For this review, take the finished solid that the model builds, in its own axes (mm). A direction names the side the tool comes from. Coordinates: 2 decimals unless noted, no trailing zeros. Loops run counter-clockwise (first coordinate to the right, second up) from the corner with the lowest first, then second, coordinate; pieces in that order, holes last. Notation, with made-up numbers: (-22, 37) - (26, 37) arc R27 ccw to (26, 69) - close; hole circle Ø3 at (57.25, 72.25). An arc over 180 degrees is marked (long way). Answer as a JSON object with one key per item and string values. Group by question number.
Item 1: We need section C-C (x = 9). Give the boundary of the cut face in (y, z) (3 decimals).
Item 2: Tool access review of faces 5 (the cylindrical face through (4.97, -8.45, -11.02)), 6 (the cylindrical face through (0.74, 17.06, 10.88)), 7 (the flat face through (0, -4, 0)), 8 (the cylindrical face through (8.028, 12.118, 3.816)), 9 (the cylindrical face through (2, -5, 0)): name each direction out of +Z, -Z, +X, -X, +Y, -Y from which nothing blocks a thin tool from reaching the whole face with its end or side.
Item 3: Mouldability with a two-part tool opening along Y and no side actions: class faces 1 (the cylindrical face through (5, 0, 11)), 2 (the cylindrical face through (2.218, 0.867, -12.905)), 3 (the flat face through (10, -13, 0)), 4 (the conical face through (6.874, -13.856, -3.077)) as released by +Y, released by -Y, zero draft, split by the parting line, or undercut.
Item 4: To check wall thickness, follow line 1 (X direction, y = 9, z = 4.5); line 2 (Y direction, x = 9.25, z = 10.5); line 3 (X direction, y = 4, z = -14). State the ranges of each line that lie inside material, in increasing order.
Item 5: Clearance check with flat-ended pins moving along their axes: pin 1 (7 mm diameter, centred on y = 9, z = 0, fed in from -X); pin 2 (12.5 mm diameter, centred on y = -2.5, z = 2, fed in from +X); pin 3 (4 mm diameter, centred on x = 1.5, z = -8.5, fed in from -Y). State where each tip first meets the part, or that it passes through.
Item 6: We need section B-B (y = 0). State how many separate pieces and enclosed holes the cut face has, then the cut area to 3 significant figures.
Item 7: We need section A-A (x = 5.5). Give the boundary of the cut face in (y, z) (1 decimal), then the cut area to 3 significant figures.
from build123d import *

# Parameters (mm, degrees)
F2_R           = 12.705
F3_DEPTH       = 4
F5_D           = 4
F5_CBORE_D     = 8
F5_CBORE_DEPTH = 4.5
F6_R           = 1.5875
F7_DEPTH       = 10.001


with BuildPart() as f1:
    # F0 (on Front) → F1 (revolve)
    with BuildSketch(Plane.XZ):
        Polygon((0, 20.234926), (0, 0), (10, 0), (10, 20.234926), (8.4925, 20.234926), (6.791023, 13.884926), (3.208977, 13.884926), (1.5075, 20.234926), align=None)
    revolve(axis=Axis((5, 0, 0), (-1, 0, 0)))

    # F2 (on face) → F3 (cut)
    with BuildSketch(Plane.YZ.offset(10)):
        Circle(F2_R)
    extrude(amount=-F3_DEPTH, mode=Mode.SUBTRACT)

    # F5 (through all)
    with Locations(Plane(origin=(0, 0, 0), x_dir=(0, -1, 0), z_dir=(-1, 0, 0))):
        with Locations((0, 9), (-9, 0), (0, -9), (9, 0)):
            CounterBoreHole(F5_D / 2, F5_CBORE_D / 2, F5_CBORE_DEPTH)

    # F6 (on face) → F7 (cut, through all)
    with BuildSketch(Plane(origin=(0, 0, 0), x_dir=(0, -1, 0), z_dir=(-1, 0, 0))):
        Circle(F6_R)
    extrude(amount=-F7_DEPTH, mode=Mode.SUBTRACT)


solid = f1.part
Check sheet entries:
{
 "1": {"outline": "circle Ø40.47 at (0, 0); hole circle Ø25.41 at (0, 0)"},
 "2": {"face 5": "none", "face 6": "+X, -X", "face 7": "+Z, -Z, -X, +Y, -Y", "face 8": "+X", "face 9": "-X"},
 "3": {"face 1": "undercut", "face 2": "undercut", "face 3": "zero draft", "face 4": "split by the parting line"},
 "4": {"line 1": "x = 0 to 6", "line 2": "y = -17.3 to -7.15, 7.15 to 17.3", "line 3": "x = 0 to 3.03, 6.97 to 10"},
 "5": {"pin 1": "stops at x = 4.5", "pin 2": "stops at x = 6", "pin 3": "stops at y = -19.16"},
 "6": {"separate pieces": "4", "enclosed holes": "0", "area": "133 mm2"},
 "7": {"outline": "circle Ø27.8 at (0, 0); hole circle Ø4 at (-9, 0); hole circle Ø4 at (0, -9); hole circle Ø4 at (0, 9); hole circle Ø3.2 at (0, 0); hole circle Ø4 at (9, 0)", "area": "547 mm2"}
}
